Work out the finished part from the listing and answer in its coordinate system (mm). Face numbers are marked on the shaded views. A direction names the side the tool comes from. Round coordinates to 2 decimals unless told otherwise and drop trailing zeros. Order: outer loops, then holes, each group sorted by start corner. A loop starts at its lowest first (then second) coordinate and runs counter-clockwise, first axis right, second up. Notation, with made-up numbers: (-19, 6.5) - (12, 6.5) arc R14 cw to (12, 30.5) - close; hole circle Ø8 at (49.25, 9). An arc over 180 degrees is marked (long way). Put each result on its own line as item: value.
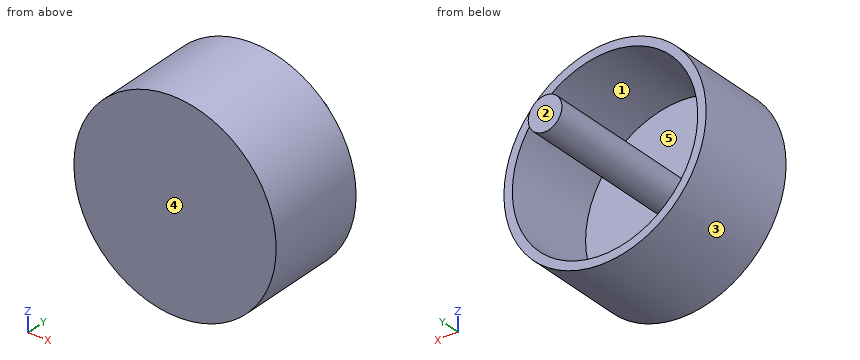
```python
from build123d import *

# Parameters (mm, degrees)
SKETCH1_R           = 76.2
BOSS_EXTRUDE1_DEPTH = 76.2
SKETCH2_R           = 12.7
BOSS_EXTRUDE2_DEPTH = 57.15
SKETCH3_R           = 69.85
SKETCH3_R_2         = 12.7
CUT_EXTRUDE1_DEPTH  = 69.85


with BuildPart() as part:
    # Sketch1 → Boss-Extrude1 (new body)
    with BuildSketch(Plane(origin=(0, 0, 0), x_dir=(1, 0, 0), z_dir=(0, 1, 0))):
        Circle(SKETCH1_R)
    extrude(amount=BOSS_EXTRUDE1_DEPTH)

    # Sketch2 → Boss-Extrude2 (add)
    with BuildSketch(Plane(origin=(0, 76.2, 0), x_dir=(1, 0, 0), z_dir=(0, 1, 0))):
        Circle(SKETCH2_R)
    extrude(amount=BOSS_EXTRUDE2_DEPTH)

    # Sketch3 → Cut-Extrude1 (cut)
    with BuildSketch(Plane(origin=(0, 76.2, 0), x_dir=(1, 0, 0), z_dir=(0, 1, 0))):
        Circle(SKETCH3_R)
        Circle(SKETCH3_R_2, mode=Mode.SUBTRACT)
    extrude(amount=-CUT_EXTRUDE1_DEPTH, mode=Mode.SUBTRACT)


solid = part.part
```
1) For a pull along X with two mould halves and no side action, classify the marked faces 3, 4 and 5 as pulls with the +X half, pulls with the -X half, needs draft (parallel to the pull), parting line crosses it, or undercut.
Findings below:
face 3: parting line crosses it
face 4: needs draft
face 5: undercut
2) Straight lines are drawn through the part: L1, parallel to Z at x = 0, y = 45; L2, parallel to Z at x = -6, y = 63.5. For each, find the intervals that lie inside material, in ascending order. Write a range as from..to.
Findings below:
L1: z = -76.2..-69.85, -12.7..12.7, 69.85..76.2
L2: z = -75.96..-69.59, -11.19..11.19, 69.59..75.96
3) For the marked faces 1 and 2, determine the directions among +Z, -Z, +X, -X, +Y, -Y from which every point of the face is accessible in a straight line to the end or side of a thin tool.
Findings below:
face 1: +Y
face 2: +Z, -Z, +X, -X, +Y
4) A cutting plane is placed at D-D on y = 97.5. Write down the section's boundary in (x, z).
Findings below:
outline: circle Ø25.4 at (0, 0)
5) A cutting plane is placed at B-B on y = 17. Write down the section's boundary in (x, z), then the cut area to 3 significant figures.
Findings below:
outline: circle Ø152.4 at (0, 0); circle Ø25.4 at (0, 0); hole circle Ø139.7 at (0, 0)
area: 3,420 mm2
6) A cutting plane is placed at C-C on x = 0. Write down the section's boundary in (y, z).
Findings below:
outline: (0, -76.2) - (76.2, -76.2) - (76.2, -69.85) - (6.35, -69.85) - (6.35, -12.7) - (133.35, -12.7) - (133.35, 12.7) - (6.35, 12.7) - (6.35, 69.85) - (76.2, 69.85) - (76.2, 76.2) - (0, 76.2) - close
7) A cutting plane is placed at A-A on z = 0. Write down the section's boundary in (x, y), then the cut area to 3 significant figures.
Findings below:
outline: (-76.2, 0) - (76.2, 0) - (76.2, 76.2) - (69.85, 76.2) - (69.85, 6.35) - (12.7, 6.35) - (12.7, 133.35) - (-12.7, 133.35) - (-12.7, 6.35) - (-69.85, 6.35) - (-69.85, 76.2) - (-76.2, 76.2) - close
area: 5,080 mm2
8) Given pin 1 Ø4 at (x, y) = (-35, 75) entering from +Z; pin 2 Ø5 at (x, y) = (22, 35) entering from -Z; pin 3 Ø3 at (x, z) = (24.5, 52.5) entering from +Y, each flat-ended and moving along its own axis, determine where each tip first touches the part or whether it passes through.
Findings below:
pin 1: stops at z = 68.68
pin 2: stops at z = -73.66
pin 3: stops at y = 6.35
